```python
from build123d import *

# Parameters (mm, degrees)
BOSS_EXTRUDE1_DEPTH = 45
SKETCH4_R           = 1.65
CUT_EXTRUDE1_DEPTH  = 7
CUT_EXTRUDE2_DEPTH  = 1.5


with BuildPart() as part:
    # Sketch1 → Boss-Extrude1 (new body)
    with BuildSketch(Plane.XY):
        Polygon((-21.15, 17.260912703), (-17.260912703, 21.15), (17.260912703, 21.15), (21.15, 17.260912703), (21.15, -17.260912703), (17.260912703, -21.15), (-17.260912703, -21.15), (-21.15, -17.260912703), align=None)
    extrude(amount=BOSS_EXTRUDE1_DEPTH)

    # Sketch3 → Revolve1 (revolve)
    with BuildSketch(Plane(origin=(0, 0, 0), x_dir=(0, 0, -1), z_dir=(1, 0, 0))):
        Polygon((-45, 21.15), (-87.3, 21.15), (-87.3, 12.5), (-89.3, 12.5), (-89.3, 4), (-110.8, 4), (-110.8, 0), (-45, 0), align=None)
    revolve(axis=Axis((0, 0, 110.8), (0, 0, -1)))

    # Sketch4 → Cut-Extrude1 (cut)
    with BuildSketch(Plane.XY.offset(87.3)):
        with Locations((0, 17.5)):
            Circle(SKETCH4_R)
        with Locations((17.5, 0)):
            Circle(SKETCH4_R)
        with Locations((0, -17.5)):
            Circle(SKETCH4_R)
        with Locations((-17.5, 0)):
            Circle(SKETCH4_R)
    extrude(amount=-CUT_EXTRUDE1_DEPTH, mode=Mode.SUBTRACT)

    # Sketch5 → Cut-Extrude2 (cut)
    with BuildSketch(Plane(origin=(4, 0, 0), x_dir=(0, 0, -1), z_dir=(1, 0, 0))):
        with BuildLine():
            Line((-106.7, 1.5), (-95.7, 1.5))
            ThreePointArc((-95.7, 1.5), (-94.2, 0), (-95.7, -1.5))
            Line((-95.7, -1.5), (-106.7, -1.5))
            ThreePointArc((-106.7, -1.5), (-108.2, 0), (-106.7, 1.5))
        make_face()
    extrude(amount=-CUT_EXTRUDE2_DEPTH, mode=Mode.SUBTRACT)


solid = part.part
```
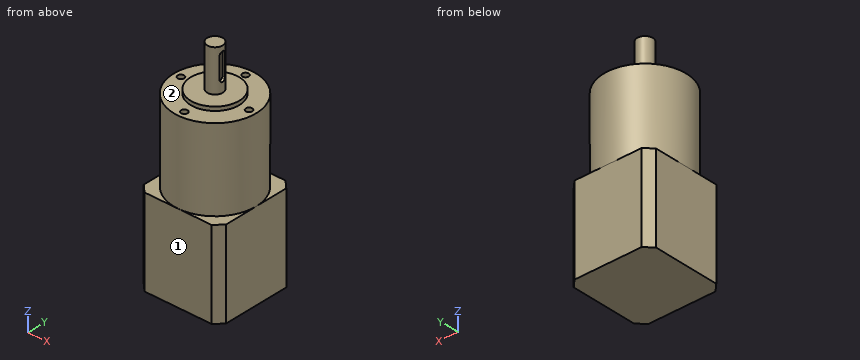
Design review of the part built by this model. Coordinates are the model's own, in mm. Face numbers are marked on the shaded views. A direction names the side the tool comes from. Give positions to 0.01 mm unless a question says otherwise; leave off trailing zeros. Order: outer loops, then holes, each group sorted by start corner. A loop starts at its lowest first (then second) coordinate and runs counter-clockwise, first axis right, second up. Notation, with made-up numbers: (76, -19) - (81, -19) arc R21 ccw to (81, -5) - close; hole circle Ø7 at (-14.5, -35.5). An arc over 180 degrees is marked (long way). Use a Markdown table: item, result. Add a question column.
(1) Add section A-A on z = 39. Give the boundary of the cut face in (x, y), then the cut area to 3 significant figures.
(2) Add section C-C on z = 92.5. Give the boundary of the cut face in (x, y).
(3) Add section D-D on z = 71. Give the boundary of the cut face in (x, y), then the cut area to 3 significant figures.
(4) Clearance check with flat-ended pins moving along their axes: P1, Ø5, axis at x = 2, z = 73, coming from the +Y side; P2, Ø5.5, axis at x = 17.5, y = 0, coming from the +Z side; P3, Ø17, axis at x = 14, y = -12.5, coming from the +Z side; P4, Ø2.5, axis at x = 0, y = -17.5, coming from the +Z side. State where each tip first meets the part, or that it passes through.
(5) Wall thickness on probe 1 along Z at (x, y) = (-8, -6); probe 2 along Z at (x, y) = (-17, 13); probe 3 along X at (y, z) = (17, 83): over which ranges is each line inside the solid? List them lowest first. Write a range as [from, to].
(6) Machinability: for the marked faces 1 and 2, which of the approach directions +Z, -Z, +X, -X, +Y, -Y give a long, thin tool a straight path to every point of the face, cutting with its end or side? Answer none if there is none.
(7) Add section B-B on y = -7.5. Give the boundary of the cut face in (x, z), then the cut area to 3 significant figures.
Report:
| question | item | result |
|---|---|---|
| 1 | outline | (-21.15, -17.26) - (-17.26, -21.15) - (17.26, -21.15) - (21.15, -17.26) - (21.15, 17.26) - (17.26, 21.15) - (-17.26, 21.15) - (-21.15, 17.26) - close |
| 1 | area | 1,760 mm² |
| 2 | outline | circle Ø8 at (0, 0) |
| 3 | outline | circle Ø42.3 at (0, 0) |
| 3 | area | 1,410 mm² |
| 4 | P1 | stops at y = 21.15 |
| 4 | P2 | stops at z = 87.3 |
| 4 | P3 | stops at z = 89.3 |
| 4 | P4 | stops at z = 80.3 |
| 5 | probe 1 | z = [0, 89.3] |
| 5 | probe 2 | z = [0, 45] |
| 5 | probe 3 | x = [-12.58, -1.57], [1.57, 12.58] |
| 6 | face 1 | +Z, -Z, +X, -X, -Y |
| 6 | face 2 | +Z |
| 7 | outline | (-21.15, 0) - (21.15, 0) - (21.15, 45) - (19.78, 45) - (19.78, 87.3) - (10, 87.3) - (10, 89.3) - (-10, 89.3) - (-10, 87.3) - (-19.78, 87.3) - (-19.78, 45) - (-21.15, 45) - close |
| 7 | area | 3,620 mm² |
